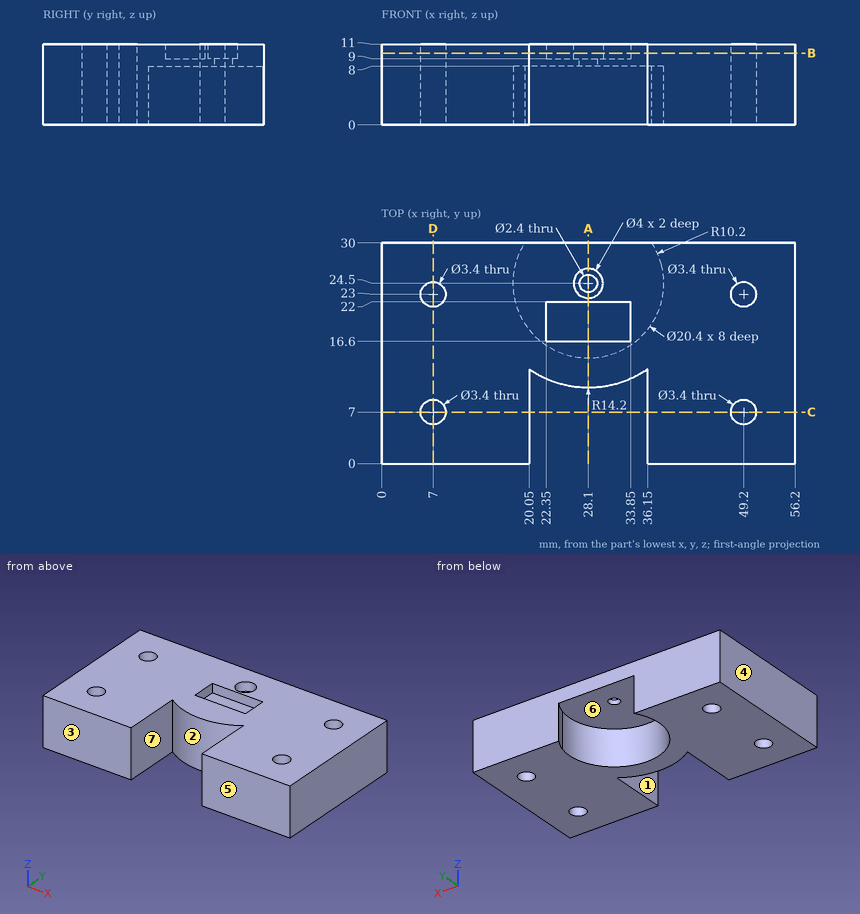
Geometry check sheet. Reference: drawing and pictorial views, mm from the part's lowest x, y, z. A direction names the side the tool comes from. Coordinates: 2 decimals unless noted, no trailing zeros. Write each loop counter-clockwise with the first axis right and the second up, starting at its lowest first coordinate (ties: lowest second). Pieces come first, ordered by that corner, then holes. Notation, with made-up numbers: M 49.25,11.25 L 104.25,11.25 A14 ccw 104.25,21.25 Z; hole C -26.75,26.25 d10. An arc over 180 degrees is marked long. Use one line per item in the form item = value.
Item 1: Release check for a two-part mould opening along X. For the marked faces 1, 2, 3 and 4 record: pulls with the +X half, pulls with the -X half, needs draft (parallel to the pull), parting line crosses it, or undercut.
Answer below:
face_1 = undercut
face_2 = undercut
face_3 = needs draft
face_4 = pulls with the -X half
Item 2: Sectioned sample at C-C, the plane y = 7. Record the cut outline in (x, z).
Answer below:
outline = M 0,0 L 5.3,0 L 5.3,11 L 0,11 Z; M 8.7,0 L 20.05,0 L 20.05,11 L 8.7,11 Z; M 36.15,0 L 47.5,0 L 47.5,11 L 36.15,11 Z; M 50.9,0 L 56.2,0 L 56.2,11 L 50.9,11 Z
Item 3: Material ranges on L1, parallel to Y at x = 49.2, z = 7.75; L2, parallel to Y at x = 28.1, z = 10.45; L3, parallel to X at y = 11.75, z = 5.25, recorded low to high. Write a range as from..to.
Answer below:
L1 = 0..5.3, 8.7..21.3, 24.7..30
L2 = 10.3..16.6, 22..22.5, 26.5..30
L3 = 0..20.05, 21.85..34.35, 36.15..56.2
Item 4: Set-up check for the marked faces 5, 6 and 7: record each of +Z, -Z, +X, -X, +Y, -Y from which the full face is reachable in a straight line by a thin tool's end or side.
Answer below:
face_5 = +Z, -Z, +X, -X, -Y
face_6 = -Z
face_7 = +Z, -Z, -Y
Item 5: Gauge pin test, flat ends, axial feed: pin 1 Ø0.6 at (x, z) = (28, 10.5) entering from -Y; pin 2 Ø3 at (x, y) = (28.1, 24.5) entering from -Z; pin 3 Ø1.5 at (x, y) = (22, 10) entering from +Z. Record the tip position at first contact, or that the pin passes through.
Answer below:
pin_1 = 10.3
pin_2 = 8
pin_3 = through
Item 6: Sectioned sample at B-B, the plane z = 9.75. Record the cut outline in (x, y).
Answer below:
outline = M 0,0 L 20.05,0 L 20.05,12.8 A14.2 ccw 36.15,12.8 L 36.15,0 L 56.2,0 L 56.2,30 L 0,30 Z; hole C 7,7 d3.4; hole C 7,23 d3.4; hole M 22.35,16.6 L 33.85,16.6 L 33.85,22 L 22.35,22 Z; hole C 28.1,24.5 d4; hole C 49.2,7 d3.4; hole C 49.2,23 d3.4
Item 7: Sectioned sample at D-D, the plane x = 7. Record the cut outline in (y, z).
Answer below:
outline = M 0,0 L 5.3,0 L 5.3,11 L 0,11 Z; M 8.7,0 L 21.3,0 L 21.3,11 L 8.7,11 Z; M 24.7,0 L 30,0 L 30,11 L 24.7,11 Z
Item 8: Sectioned sample at A-A, the plane x = 28.1. Record the cut outline in (y, z), and give its area (3 significant figures).
Answer below:
outline = M 10.3,0 L 14.3,0 L 14.3,8 L 23.3,8 L 23.3,9 L 22.5,9 L 22.5,11 L 22,11 L 22,9 L 16.6,9 L 16.6,11 L 10.3,11 Z; M 25.7,8 L 30,8 L 30,11 L 26.5,11 L 26.5,9 L 25.7,9 Z
area = 69.9 mm^2
